Geometry: see drawing. Coordinates: mm, zero at the bounding-box minimum. A direction names the side the tool comes from. Give positions to 0.01 mm unless a question says otherwise; leave off trailing zeros. Loops run counter-clockwise (first coordinate to the right, second up) from the corner with the lowest first, then second, coordinate; pieces in that order, holes last. Notation, with made-up numbers: M 46,87 L 54,87 A16 ccw 54,91 Z; hole C 23,46.25 d11. An arc over 180 degrees is marked long. Put each result on its own line as item: value.
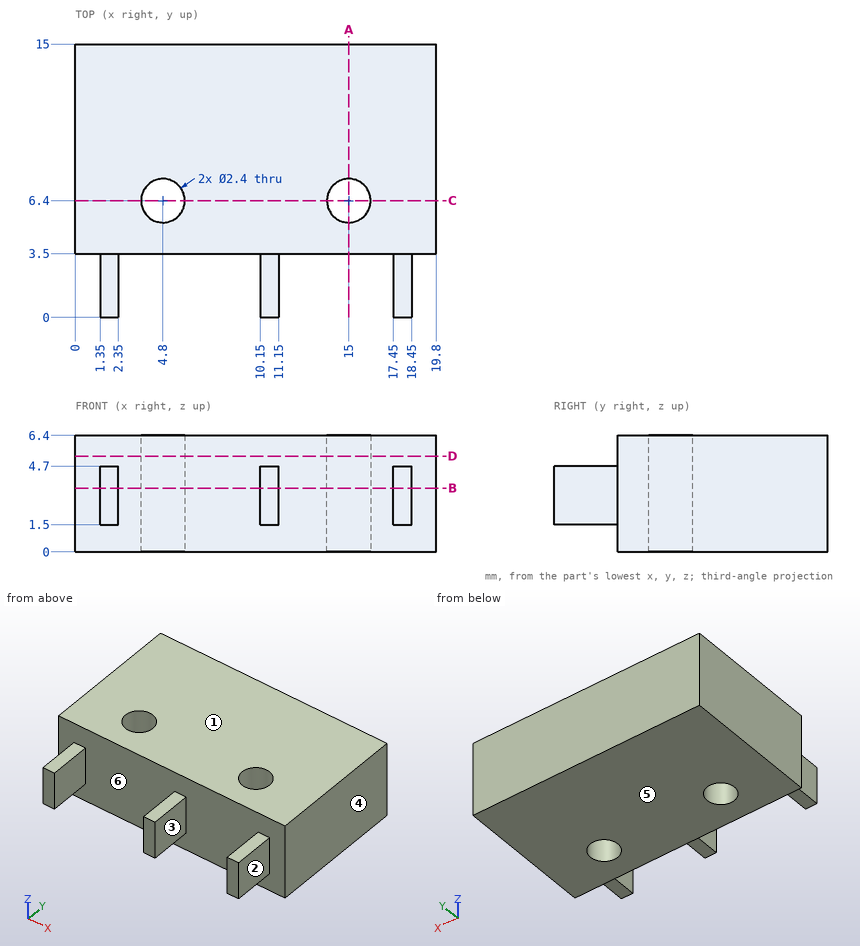
1. Access query for the marked faces 1, 2 and 3. Directions: +Z, -Z, +X, -X, +Y, -Y. A direction counts if a zero-diameter tool reaches every point of the face in a straight line with its end or side. Return the directions, or none.
Found:
face 1: +Z, +X, -X, +Y, -Y
face 2: +Z, -Z, +X, -Y
face 3: +Z, -Z, -Y
2. Draft query along X for the marked faces 4, 5 and 6. Return one class per face: pulls with the +X half, pulls with the -X half, needs draft (parallel to the pull), parting line crosses it, or undercut.
Found:
face 4: pulls with the +X half
face 5: needs draft
face 6: undercut
3. Section query B-B (z = 3.5). Output: boundary loops of the cut face in (x, y).
Found:
outline: M 0,3.5 L 1.35,3.5 L 1.35,0 L 2.35,0 L 2.35,3.5 L 10.15,3.5 L 10.15,0 L 11.15,0 L 11.15,3.5 L 17.45,3.5 L 17.45,0 L 18.45,0 L 18.45,3.5 L 19.8,3.5 L 19.8,15 L 0,15 Z; hole C 4.8,6.4 d2.4; hole C 15,6.4 d2.4
4. Section query D-D (z = 5.25). Output: boundary loops of the cut face in (x, y), plus the area to 3 significant figures.
Found:
outline: M 0,3.5 L 19.8,3.5 L 19.8,15 L 0,15 Z; hole C 4.8,6.4 d2.4; hole C 15,6.4 d2.4
area: 219 mm^2
5. Section query A-A (x = 15). Output: boundary loops of the cut face in (y, z), plus the area to 3 significant figures.
Found:
outline: M 3.5,0 L 5.2,0 L 5.2,6.4 L 3.5,6.4 Z; M 7.6,0 L 15,0 L 15,6.4 L 7.6,6.4 Z
area: 58.2 mm^2
6. Contact query for flat-ended pins moving along their axis: P1, Ø1, axis at y = 1.5, z = 2.5, coming from the -X side; P2, Ø2.5, axis at y = 2, z = 3.5, coming from the +X side; P3, Ø3.5, axis at y = 2.5, z = 3.5, coming from the -X side; P4, Ø1.1, axis at x = 18, y = 2.5, coming from the +Z side. Output: stop coordinate, or through.
Found:
P1: x = 1.35
P2: x = 18.45
P3: x = 0
P4: z = 4.7
7. Material intervals for line 1 (Y direction, x = 15, z = 4); line 2 (X direction, y = 7.25, z = 5.5); line 3 (X direction, y = 6, z = 1), sorted ascending. Write a range as from..to.
Found:
line 1: 3.5..5.2, 7.6..15
line 2: 0..3.95, 5.65..14.15, 15.85..19.8
line 3: 0..3.67, 5.93..13.87, 16.13..19.8
8. Section query C-C (y = 6.4). Output: boundary loops of the cut face in (x, z).
Found:
outline: M 0,0 L 3.6,0 L 3.6,6.4 L 0,6.4 Z; M 6,0 L 13.8,0 L 13.8,6.4 L 6,6.4 Z; M 16.2,0 L 19.8,0 L 19.8,6.4 L 16.2,6.4 Z
